Can you work these out from the drawing? Everything is in mm from the part's minimum corner. A direction names the side the tool comes from. Round coordinates to 2 decimals unless told otherwise and drop trailing zeros. Write each loop counter-clockwise with the first axis right and the second up, starting at its lowest first coordinate (ties: lowest second). Pieces come first, ordered by that corner, then holes. Notation, with made-up numbers: (52.5, 52) -> (79.5, 52) arc R29 cw to (79.5, 86) -> close; hole circle Ø2 at (-13.75, -9.75). An arc over 180 degrees is marked (long way). Put each result on its own line as item: value. Start each with the question number.
1. I need wall thicknesses on probe 1 along Y at (x, z) = (70, 16); probe 2 along Z at (x, y) = (23.5, 41.5); probe 3 along X at (y, z) = (34.5, 18). Which ranges of each line are inside material? Lowest first, please. Write a range as from..to.
2. Suppose I cut it at A-A (y = 56). Please give me the cut outline in (x, z), then the cut area to 3 significant figures.
3. Suppose I cut it at C-C (z = 6.5). Please give me the cut outline in (x, y).
4. Suppose I cut it at B-B (x = 75.5). Please give me the cut outline in (y, z), then the cut area to 3 significant figures.
5. Suppose I cut it at D-D (x = 30). Please give me the cut outline in (y, z), then the cut area to 3 significant figures.
6. Which directions (+Z, -Z, +X, -X, +Y, -Y) give clear straight access to the entire face, cutting with the end or side of a thin tool? Please do the marked faces 4, 5 and 6.
7. We'd pull the mould along Y, two halves only. Please class the marked faces 1, 2 and 3: +Y half, -Y half, draft (parallel to the pull), parting line (faces both ways), or undercut.
8. For pin 1 (8 mm diameter, centred on y = 61, z = 41.5, fed in from +X); pin 2 (25 mm diameter, centred on x = 70, y = 42, fed in from +Z); pin 3 (1 mm diameter, centred on x = 87.5, y = 75, fed in from +Z); pin 4 (3 mm diameter, centred on y = 58.5, z = 19.5, fed in from +X), each with a flat end and sliding along its axis, tell me the tip position at first contact or that it passes through.
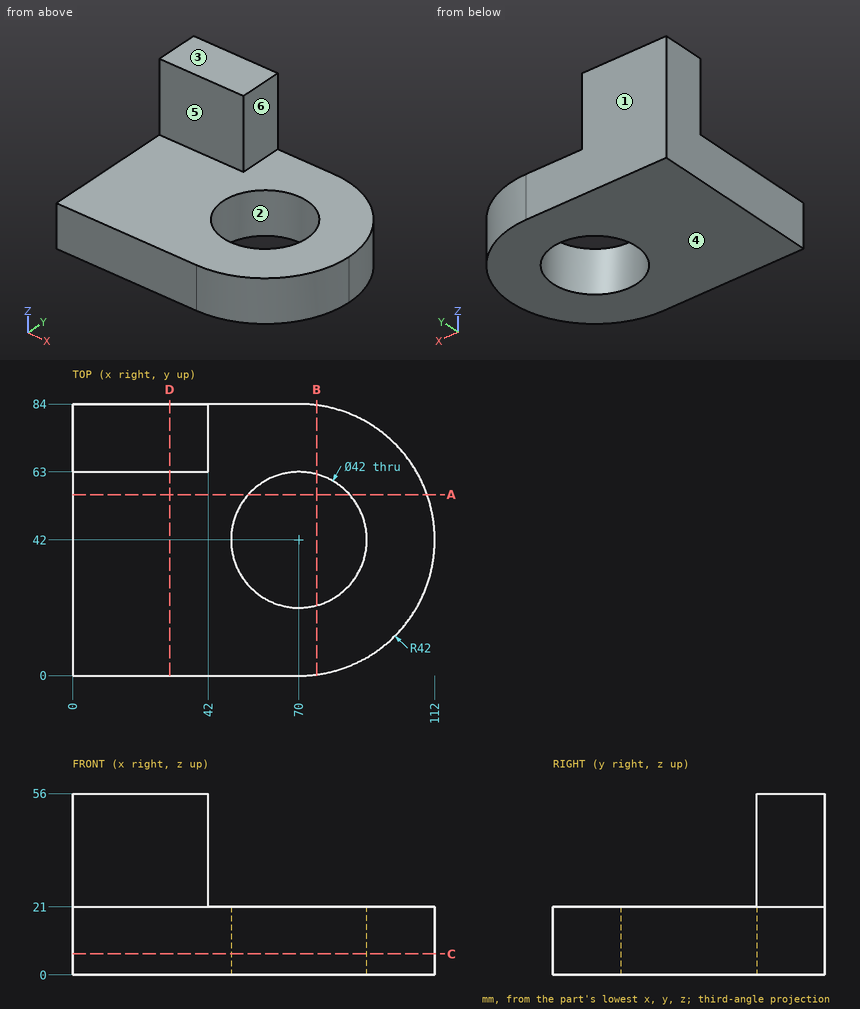
Verdict:
1. probe 1: y = 0..21, 63..84
1. probe 2: z = 0..21
1. probe 3: x = 0..50.38, 89.62..111.32
2. outline: (0, 0) -> (54.35, 0) -> (54.35, 21) -> (0, 21) -> close; (85.65, 0) -> (109.6, 0) -> (109.6, 21) -> (85.65, 21) -> close
2. area: 1,640 mm^2
3. outline: (0, 0) -> (70, 0) arc R42 ccw to (112, 42) arc R42 ccw to (70, 84) -> (0, 84) -> close; hole circle Ø42 at (70, 42)
4. outline: (0.36, 0) -> (21.73, 0) -> (21.73, 21) -> (0.36, 21) -> close; (62.27, 0) -> (83.64, 0) -> (83.64, 21) -> (62.27, 21) -> close
4. area: 898 mm^2
5. outline: (0, 0) -> (84, 0) -> (84, 56) -> (63, 56) -> (63, 21) -> (0, 21) -> close
5. area: 2,500 mm^2
6. face 4: -Z, +X, -X, +Y, -Y
6. face 5: +Z, +X, -X, -Y
6. face 6: +Z, +X, +Y, -Y
7. face 1: +Y half
7. face 2: undercut
7. face 3: draft
8. pin 1: stops at x = 42
8. pin 2: passes through
8. pin 3: stops at z = 21
8. pin 4: stops at x = 109.23
